```python
from build123d import *

# Parameters (mm, degrees)
SKETCH1_R               = 18.415
BOSS_EXTRUDE2_DEPTH     = 113.03
SKETCH4_W               = 20.32
SKETCH4_H               = 5.08
CUT_EXTRUDE2_DEPTH      = 12.7
CUT_EXTRUDE2_DEPTH_BACK = 22.86
CUT_EXTRUDE3_START      = -5.08
SKETCH5_R               = 13.462
CUT_EXTRUDE3_DEPTH      = 107.95


with BuildPart() as part:
    # Sketch1 → Boss-Extrude2 (new body)
    with BuildSketch(Plane.XY):
        Circle(SKETCH1_R)
    extrude(amount=BOSS_EXTRUDE2_DEPTH)

    # Sketch4 → Cut-Extrude2 (cut, two sides)
    with BuildSketch(Plane(origin=(0, 0, 0), x_dir=(1, 0, 0), z_dir=(0, 1, 0))) as cut_extrude2_sk:
        with Locations((0, -106.68)):
            Rectangle(SKETCH4_W, SKETCH4_H)
    extrude(amount=CUT_EXTRUDE2_DEPTH, mode=Mode.SUBTRACT)
    extrude(cut_extrude2_sk.sketch, amount=-CUT_EXTRUDE2_DEPTH_BACK, mode=Mode.SUBTRACT)

    # Sketch5 → Cut-Extrude3 (cut)
    with BuildSketch(Plane(origin=(0, 0, 0), x_dir=(-1, 0, 0), z_dir=(0, 0, -1)).offset(CUT_EXTRUDE3_START)):
        Circle(SKETCH5_R)
    extrude(amount=-CUT_EXTRUDE3_DEPTH, mode=Mode.SUBTRACT)


solid = part.part
```
Read the model definition and answer for the solid it produces. Units are mm, in the model's axes. A direction names the side the tool comes from. Coordinates: 2 decimals unless noted, no trailing zeros. Loops run counter-clockwise (first coordinate to the right, second up) from the corner with the lowest first, then second, coordinate; pieces in that order, holes last.
(1) The part is cut by section A-A (x = 0). Determine the outline of the cut face in (y, z) (3 decimals), and give its area (3 significant figures).
Solution:
outline: (-18.415, 0) - (18.415, 0) - (18.415, 113.03) - (13.462, 113.03) - (13.462, 5.08) - (-13.462, 5.08) - (-13.462, 104.14) - (-18.415, 104.14) - close; (-18.415, 109.22) - (-13.462, 109.22) - (-13.462, 113.03) - (-18.415, 113.03) - close
area: 1,230 mm2
(2) The part is cut by section B-B (y = 0). Determine the outline of the cut face in (x, z) (3 decimals).
Solution:
outline: (-18.415, 0) - (18.415, 0) - (18.415, 113.03) - (13.462, 113.03) - (13.462, 5.08) - (-13.462, 5.08) - (-13.462, 113.03) - (-18.415, 113.03) - close
(3) The part is cut by section D-D (x = 9). Determine the outline of the cut face in (y, z).
Solution:
outline: (-16.07, 0) - (16.07, 0) - (16.07, 113.03) - (10.01, 113.03) - (10.01, 109.22) - (12.7, 109.22) - (12.7, 104.14) - (10.01, 104.14) - (10.01, 5.08) - (-10.01, 5.08) - (-10.01, 104.14) - (-16.07, 104.14) - close; (-16.07, 109.22) - (-10.01, 109.22) - (-10.01, 113.03) - (-16.07, 113.03) - close
(4) The part is cut by section C-C (z = 31). Determine the outline of the cut face in (x, y) (3 decimals), and give its area (3 significant figures).
Solution:
outline: circle Ø36.83 at (0, 0); hole circle Ø26.924 at (0, 0)
area: 496 mm2
(5) A tool of negligible diameter and unlimited length cuts with its end or side. For faces 1 (the face through (0, 0, 0)), 2 (the face through (7, 12.7, 107)), 3 (the face through (0, 0, 5.08)), from which of +Z, -Z, +X, -X, +Y, -Y can it reach the whole face along a straight path? Write none if from no direction.
Solution:
face 1: -Z, +X, -X, +Y, -Y
face 2: -Y
face 3: +Z
(6) Consider line 1 along Y through (x, z) = (0, 78) (3 decimals); line 2 along Z through (x, y) = (8.5, 11); line 3 along Z through (x, y) = (3, 3). Determine where each line is inside the solid, lowest interval first.
Solution:
line 1: y = -18.415 to -13.462, 13.462 to 18.415
line 2: z = 0 to 104.14, 109.22 to 113.03
line 3: z = 0 to 5.08
(7) Flat-ended cylindrical pins translate along their axes: pin 1 Ø1 at (y, z) = (-4, 77) entering from +X; pin 2 Ø5.5 at (x, z) = (-8, 106.5) entering from -Y; pin 3 Ø1.5 at (x, z) = (-6, 68.5) entering from +Y; pin 4 Ø3 at (x, y) = (-2.5, -12) entering from -Z. Find the tip coordinate at first contact, or state that the pin passes through.
Solution:
pin 1: stops at x = 18.08
pin 2: stops at y = -17.2
pin 3: stops at y = 17.65
pin 4: stops at z = 0
(8) The mould has two halves that part along Y. Classify faces 4 (the face through (1.752, 13.347, 58.299)), 5 (the face through (-7, 12.7, 107)), 6 (the face through (0, -15, 109.22)): released by +Y, released by -Y, zero draft, split by the parting line, or undercut.
Solution:
face 4: undercut
face 5: released by -Y
face 6: zero draft
